Here's how the part is built. I have some questions about the finished solid (model axes, mm). Coordinates: 2 decimals unless noted, no trailing zeros. Loops run counter-clockwise (first coordinate to the right, second up) from the corner with the lowest first, then second, coordinate; pieces in that order, holes last. Notation, with made-up numbers: (70.25, -13.75) -> (118.25, -13.75) arc R36 ccw to (118.25, 21.25) -> close; hole circle Ø5 at (77, -9). An arc over 180 degrees is marked (long way). Answer as a JSON object with one key per item and string values. Group by question number.
Q1. I want a section at C-C on z = 165. Write out the boundary of the cut face in (x, y), then the cut area to 3 significant figures.
Q2. I want a section at D-D on x = -56. Count the separate pieces of the cut face and the enclosed holes in it, then the cut area to 3 significant figures.
Q3. I need wall thicknesses on line 1 (Z direction, x = 156, y = -1.7); line 2 (X direction, y = -0.8, z = 3); line 3 (X direction, y = -2.75, z = 215.5). Which ranges of each line are inside material? Lowest first, please.
Q4. I want a section at B-B on x = 76.5. Write out the boundary of the cut face in (y, z), then the cut area to 3 significant figures.
Q5. I'm going to push a flat-ended pin straight in: pin 1 (2 mm diameter, centred on x = -90.5, z = -59.5, fed in from +Y). Where does the tip first touch, or does it pass through?
Q6. I want a section at A-A on z = -7.5. Write out the boundary of the cut face in (x, y).
```python
from build123d import *

# Parameters (mm, degrees)
F0_W     = 406.4
F0_H     = 508
F0_W_2   = 244.0329119563
F0_H_2   = 54.9797415733
F0_W_3   = 30.9118032455
F0_H_3   = 91.8955244124
F0_W_4   = 50.8
F0_H_4   = 38.1
F0_W_5   = 194.1293792814
F0_H_5   = 82.4762731791
F0_W_6   = 36.3956689835
F0_H_6   = 20.4090550542
F1_DEPTH = 5.08
F2_SIZE  = 5.07999


# Not quite as in the source:
# - a fillet or chamfer is up to 0.001 mm smaller than in the source, because OpenCascade refuses the exact size


with BuildPart() as f1:
    # F0 (on Front) → F1 (new body)
    with BuildSketch(Plane.XZ):
        with Locations((0.8964706212, 86.9385877169)):
            Rectangle(F0_W, F0_H)
        with Locations((-38.650367409, -116.3898707867)):
            Rectangle(F0_W_2, F0_H_2, mode=Mode.SUBTRACT)
        with Locations((142.4559016228, 20.3487034887)):
            Rectangle(F0_W_3, F0_H_3, mode=Mode.SUBTRACT)
        with Locations((-88.9, 171.45)):
            Rectangle(F0_W_4, F0_H_4, mode=Mode.SUBTRACT)
        with Locations((-42.6353103593, 244.4381365895)):
            Rectangle(F0_W_5, F0_H_5, mode=Mode.SUBTRACT)
        with Locations((3.6293792814, 171.45)):
            Rectangle(F0_W_4, F0_H_4, mode=Mode.SUBTRACT)
        with Locations((140.1178344917, 219.6642868221)):
            Rectangle(F0_W_6, F0_H_6, mode=Mode.SUBTRACT)
    extrude(amount=F1_DEPTH)

    # F2 (size 5.08 in the source; OpenCascade refuses exactly that, so slightly less here)
    f2_edges = [f1.edges().sort_by_distance(p)[0] for p in [
        (-139.7, -5.08, 244.438137),
        (-42.63531, -5.08, 285.676273),
        (54.429379, -5.08, 244.438137),
        (-42.63531, -5.08, 203.2),
    ]]
    chamfer(f2_edges, length=F2_SIZE)


solid = f1.part
```
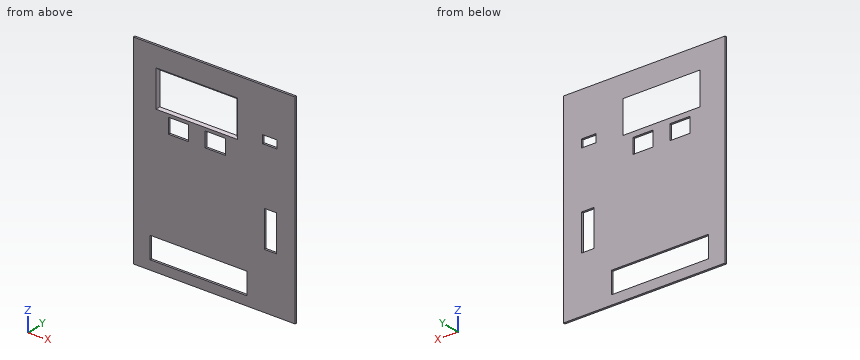
Result set:
{
 "1": {"outline": "(-202.3, -5.08) -> (-114.3, -5.08) -> (-114.3, 0) -> (-202.3, 0) -> close; (-63.5, -5.08) -> (-21.77, -5.08) -> (-21.77, 0) -> (-63.5, 0) -> close; (29.03, -5.08) -> (204.1, -5.08) -> (204.1, 0) -> (29.03, 0) -> close", "area": "1,550 mm²"},
 "2": {"separate pieces": "3", "enclosed holes": "0", "area": "1,860 mm²"},
 "3": {"line 1": "z = -167.06 to -25.6, 66.3 to 209.46, 229.87 to 340.94", "line 2": "x = -202.3 to 127, 157.91 to 204.1", "line 3": "x = -202.3 to -142.45, 57.18 to 121.92, 158.32 to 204.1"},
 "4": {"outline": "(-5.08, -167.06) -> (0, -167.06) -> (0, -143.88) -> (-5.08, -143.88) -> close; (-5.08, -88.9) -> (0, -88.9) -> (0, 340.94) -> (-5.08, 340.94) -> close", "area": "2,300 mm²"},
 "5": {"pin 1": "stops at y = 0"},
 "6": {"outline": "(-202.3, -5.08) -> (127, -5.08) -> (127, 0) -> (-202.3, 0) -> close; (157.91, -5.08) -> (204.1, -5.08) -> (204.1, 0) -> (157.91, 0) -> close"}
}
